Autodesk Inventor part; units mm, degrees
ref_plane "YZ Plane" through (0, 0, 0) normal (1, 0, 0) x (0, 1, 0)
ref_plane "XZ Plane" through (0, 0, 0) normal (0, 1, 0) x (-1, 0, 0)
ref_plane "XY Plane" through (0, 0, 0) normal (0, 0, 1) x (1, 0, 0)
sketch "Sketch2" plane through (0, 0, 0) normal (0, 1, 0) x (-1, 0, 0)
  line L0 (-7.5, 0.85) -> (-7.5, -0.85)
  line L1 (1, -2.5) -> (5, -2.5)
  line L2 (7.5, 2.5) -> (-7.5, -2.5) construction
  line L3 (-7.5, 2.5) -> (7.5, -2.5) construction
  arc A0 (5, -2.5) -> (5, 2.5) centre (5, 0) ccw
  circle A1 centre (5, 0) radius 0.9
  line L4 (-3, 0.85) -> (-7.5, 0.85)
  line L5 (-7.5, 0.85) -> (-7.5, -0.85)
  line L6 (-7.5, -0.85) -> (-3, -0.85)
  line L7 (1, 2.5) -> (-3, 0.85)
  line L8 (-3, -0.85) -> (1, -2.5)
  line L9 (5, 2.5) -> (1, 2.5)
  point P0 (0, 0)
  dimension "d3" = 1.8
extrude "Extrusion1" add sketch "Sketch2" along normal blind 0.6
sketch "Sketch3" plane through (0, 0, 0) normal (0, -1, 0) x (1, 0, 0)
  line L0 (-3.4662, 1.2021) -> (-0.4158, 1.2021) construction
  line L1 (-0.4158, 1.2021) -> (-0.4158, -1.1913) construction
  line L2 (-0.4158, -1.1913) -> (-3.4662, -1.1913) construction
  line L3 (-3.4662, -1.1913) -> (-3.4662, 1.2021) construction
  line L4 (-0.7369, -0.1589) -> (-1.7693, -0.1589)
  line L5 (-1.7693, -0.1589) -> (-1.7693, -1.1913)
  line L6 (-1.7693, -1.1913) -> (-2.1102, -1.1913)
  line L7 (-2.1102, -1.1913) -> (-2.1102, -0.1589)
  line L8 (-2.1102, -0.1589) -> (-3.1427, -0.1589)
  line L9 (-3.1427, -0.1589) -> (-3.1427, 0.1696)
  line L10 (-3.1427, 0.1696) -> (-2.1102, 0.1696)
  line L11 (-2.1102, 0.1696) -> (-2.1102, 1.2021)
  line L12 (-2.1102, 1.2021) -> (-1.7693, 1.2021)
  line L13 (-1.7693, 1.2021) -> (-1.7693, 0.1696)
  line L14 (-1.7693, 0.1696) -> (-0.7369, 0.1696)
  line L15 (-0.7369, 0.1696) -> (-0.7369, -0.1589)
  point P0 (0, 0)
extrude "Extrusion2" add sketch "Sketch3" along normal blind 0.1
properties part number "Pin" material "Copper, Alloy"
Build history of the part. All positions in model axes, mm. Coordinates: 2 decimals unless noted, no trailing zeros. Write each loop counter-clockwise with the first axis right and the second up, starting at its lowest first coordinate (ties: lowest second). Pieces come first, ordered by that corner, then holes.
1. Band-saw the part on B-B, the plane z = 0. Give the cut face in (x, y).
Answer block:
outline: (-7.5, 0) - (-5.9, 0) - (-5.9, 0.6) - (-7.5, 0.6) - close; (-4.1, 0) - (-3.14, 0) - (-3.14, -0.1) - (-0.74, -0.1) - (-0.74, 0) - (7.5, 0) - (7.5, 0.6) - (-4.1, 0.6) - close
2. Band-saw the part on A-A, the plane y = 0.35. Give the cut face in (x, z), and give its area (3 significant figures).
Answer block:
outline: (-5, -2.5) - (-1, -2.5) - (3, -0.85) - (7.5, -0.85) - (7.5, 0.85) - (3, 0.85) - (-1, 2.5) - (-5, 2.5) arc R2.5 ccw to start; hole circle Ø1.8 at (-5, 0)
area: 48.3 mm2
3. Drill centre lines: probe 1 along Z at (x, y) = (-5, 0.3); probe 2 along Y at (x, z) = (5.5, -0.6); probe 3 along Z at (x, y) = (5.25, 0.55). Where is each one in solid material? Low to high.
Answer block:
probe 1: z = -2.5 to -0.9, 0.9 to 2.5
probe 2: y = 0 to 0.6
probe 3: z = -0.85 to 0.85
4. Band-saw the part on C-C, the plane x = -2.5. Give the cut face in (y, z).
Answer block:
outline: (-0.1, -0.16) - (0, -0.16) - (0, -2.5) - (0.6, -2.5) - (0.6, 2.5) - (0, 2.5) - (0, 0.17) - (-0.1, 0.17) - close
5. Pull direction X, two halves, no side cores. Call faces 1 (the flat face through (0.972, 0.296, 1.687)), 2 (the flat face through (-1.6, 0, 0.6)), 3 (the cylindrical face through (-4.1, 0.3, 0)): released by +X, released by -X, zero draft, split by the parting line, or undercut.
Answer block:
face 1: released by +X
face 2: zero draft
face 3: undercut
6. Band-saw the part on D-D, the plane x = -4.5. Give the cut face in (y, z).
Answer block:
outline: (0, -2.5) - (0.6, -2.5) - (0.6, -0.75) - (0, -0.75) - close; (0, 0.75) - (0.6, 0.75) - (0.6, 2.5) - (0, 2.5) - close
